```python
from build123d import *

# Parameters (mm, degrees)
SKETCH1_W            = 250
SKETCH1_H            = 90
BOSS_EXTRUDE1_DEPTH  = 4
SKETCH2_R            = 3
SKETCH2_R_2          = 1.5
SKETCH2_R_3          = 2
CUT_EXTRUDE1_DEPTH   = 133.91350571
SKETCH3_R            = 2
CUT_EXTRUDE2_DEPTH   = 133.91350571
CUT_EXTRUDE3_DEPTH   = 133.91350571
FILLET1_R            = 1
FILLET1_OF_MIRROR2_R = 1
MIRROR3_OUTLINE_R    = 1.5
MIRROR3_OUTLINE_R_2  = 2
MIRROR3_DEPTH        = 4


# Read off the part's stored shape, not the designer's step: Mirror3
with BuildPart() as part:
    # Sketch1 → Boss-Extrude1 (new body)
    with BuildSketch(Plane(origin=(0, 0, 0), x_dir=(0, 0, -1), z_dir=(1, 0, 0))):
        Rectangle(SKETCH1_W, SKETCH1_H)
    extrude(amount=BOSS_EXTRUDE1_DEPTH)

    # Sketch2 → Cut-Extrude1 (cut, through all)
    with BuildSketch(Plane(origin=(4, 0, 0), x_dir=(0, 0, -1), z_dir=(1, 0, 0))):
        Circle(SKETCH2_R)
        with Locations((-48, 0)):
            Circle(SKETCH2_R_2)
        with Locations((-89, 0)):
            Circle(SKETCH2_R_3)
        with Locations((-114, 0)):
            Circle(SKETCH2_R_2)
    extrude(amount=-CUT_EXTRUDE1_DEPTH, mode=Mode.SUBTRACT)

    # Sketch3 → Cut-Extrude2 (cut, through all)
    with BuildSketch(Plane(origin=(4, 0, 0), x_dir=(0, 0, -1), z_dir=(1, 0, 0))):
        with Locations((-20, 30)):
            Circle(SKETCH3_R)
    cut_extrude2 = extrude(amount=-CUT_EXTRUDE2_DEPTH, mode=Mode.SUBTRACT)

    # Sketch4 → Cut-Extrude3 (cut, through all)
    with BuildSketch(Plane(origin=(4, 0, 0), x_dir=(0, 0, -1), z_dir=(1, 0, 0))):
        with BuildLine():
            Line((-114, 7.5), (-50, 7.5))
            Line((-50, 7.5), (-42.5, 7.5))
            ThreePointArc((-42.5, 7.5), (-31.893398282, 11.893398282), (-27.5, 22.5))
            Line((-27.5, 22.5), (-27.5, 30))
            ThreePointArc((-27.5, 30), (-20, 37.5), (-12.5, 30))
            Line((-12.5, 30), (-12.5, 10))
            ThreePointArc((-12.5, 10), (-6.934403149, 14.427891494), (0, 16.007810594))
            Line((0, 16.007810594), (0, 45))
            Line((0, 45), (-125, 45))
            Line((-125, 45), (-125, 1.99556796))
            Line((-125, 1.99556796), (-125, 0))
            Line((-125, 0), (-121.5, 0))
            ThreePointArc((-121.5, 0), (-119.303300859, 5.303300859), (-114, 7.5))
        make_face()
    cut_extrude3 = extrude(amount=-CUT_EXTRUDE3_DEPTH, mode=Mode.SUBTRACT)

    # Fillet1
    fillet1_edges = [part.edges().sort_by_distance(p)[0] for p in [
        (2, 10, 12.5),
    ]]
    fillet(fillet1_edges, radius=FILLET1_R)

    # Mirror2: Cut-Extrude2, Cut-Extrude3 across plane
    add(cut_extrude2.mirror(Plane.ZX), mode=Mode.SUBTRACT)
    add(cut_extrude3.mirror(Plane.ZX), mode=Mode.SUBTRACT)

    # Fillet1 of Mirror2
    fillet1_of_mirror2_edges = [part.edges().sort_by_distance(p)[0] for p in [
        (2, -10, 12.5),
    ]]
    fillet(fillet1_of_mirror2_edges, radius=FILLET1_OF_MIRROR2_R)

    # Mirror3 outline → Mirror3 (cut)
    with BuildSketch(Plane.YZ):
        with BuildLine():
            Line((7.5, -42.5), (7.5, -114))
            ThreePointArc((7.5, -114), (0, -121.5), (-7.5, -114))
            Line((-7.5, -114), (-7.5, -42.5))
            ThreePointArc((-7.5, -42.5), (-11.893398282, -31.893398282), (-22.5, -27.5))
            Line((-22.5, -27.5), (-30, -27.5))
            ThreePointArc((-30, -27.5), (-37.5, -20), (-30, -12.5))
            Line((-30, -12.5), (-12.530587424, -12.5))
            ThreePointArc((-12.530587424, -12.5), (-11.615120349, -11.902392887), (-11.793832546, -10.823840071))
            ThreePointArc((-11.793832546, -10.823840071), (-14.917161888, -5.807605463), (-16.007810594, 0))
            Line((-16.007810594, 0), (-45, 0))
            Line((-45, 0), (-45, -125))
            Line((-45, -125), (45, -125))
            Line((45, -125), (45, 0))
            Line((45, 0), (16.007810594, 0))
            ThreePointArc((16.007810594, 0), (14.917161888, -5.807605463), (11.793832546, -10.823840071))
            ThreePointArc((11.793832546, -10.823840071), (11.615120349, -11.902392887), (12.530587424, -12.5))
            Line((12.530587424, -12.5), (30, -12.5))
            ThreePointArc((30, -12.5), (37.5, -20), (30, -27.5))
            Line((30, -27.5), (22.5, -27.5))
            ThreePointArc((22.5, -27.5), (11.893398282, -31.893398282), (7.5, -42.5))
        make_face()
        with Locations((0, -114)):
            Circle(MIRROR3_OUTLINE_R)
        with Locations((0, -89)):
            Circle(MIRROR3_OUTLINE_R_2)
        with Locations((0, -48)):
            Circle(MIRROR3_OUTLINE_R)
        with Locations((30, -20)):
            Circle(MIRROR3_OUTLINE_R_2)
        with Locations((-30, -20)):
            Circle(MIRROR3_OUTLINE_R_2)
    extrude(amount=MIRROR3_DEPTH, mode=Mode.SUBTRACT)


solid = part.part
```
Input: part model. Units: mm. Frame: model coordinates. A direction names the side the tool comes from. Round coordinates to 2 decimals unless told otherwise and drop trailing zeros. Write each loop counter-clockwise with the first axis right and the second up, starting at its lowest first coordinate (ties: lowest second). Pieces come first, ordered by that corner, then holes. Notation, with made-up numbers: (-39, 84.5) -> (1, 84.5) arc R10 ccw to (1, 95.5) -> close; hole circle Ø1 at (-16, 25.5). An arc over 180 degrees is marked (long way). Answer as CSV lines item,"result".
1. Contact query for flat-ended pins moving along their axis: P1, Ø5, axis at y = 30, z = -20, coming from the +X side; P2, Ø2, axis at x = 2, y = -25, coming from the +Z side; P3, Ø2, axis at x = 1.5, z = -85, coming from the -Y side; P4, Ø1.2, axis at x = 1.5, y = -26, coming from the -Z side. Output: stop coordinate, or through.
Geometry says:
P1,"stops at x = 4"
P2,"stops at z = 27.5"
P3,"stops at y = -7.5"
P4,"stops at z = -27.5"
2. Ray query, L1, parallel to Z at x = 0.5, y = -22.5; L2, parallel to Z at x = 3.1, y = 29; L3, parallel to Y at x = 2.25, z = -114. Return the intervals inside material, ascending. Write a range as [from, to].
Geometry says:
L1,"z = [-27.5, -12.5], [12.5, 27.5]"
L2,"z = [-27.5, -21.73], [-18.27, -12.5], [12.5, 18.27], [21.73, 27.5]"
L3,"y = [-7.5, -1.5], [1.5, 7.5]"
3. Reachability of faces 1 (the flat face through (2, -26, -27.5)), 2 (the flat face through (2, 7.5, 79)), 3 (the flat face through (2, -26, 27.5)), 4 (the flat face through (2, 26, -27.5)), 5 (the flat face through (2, 21, 12.5)) from +Z, -Z, +X, -X, +Y, -Y: full face, straight path, thin tool, end or side. Return the list, or none.
Geometry says:
face 1,"-Z, +X, -X, -Y"
face 2,"+Z, +X, -X, +Y"
face 3,"+Z, +X, -X, -Y"
face 4,"-Z, +X, -X, +Y"
face 5,"+X, -X, +Y"
4. Section A-A (x = 2.2). Give the number of separate pieces and of enclosed holes in the cut face, plus the area to 3 significant figures.
Geometry says:
separate pieces,"1"
enclosed holes,"11"
area,"5,700 mm^2"
5. Section C-C (z = -37.5). Return the cut outline in (x, y), plus the area to 3 significant figures.
Geometry says:
outline,"(0, -8.36) -> (4, -8.36) -> (4, 8.36) -> (0, 8.36) -> close"
area,"66.9 mm^2"
6. Mould query, pull axis Z, two halves, no side actions, for faces 6 (the flat face through (2, 7.5, -78)), 7 (the cylindrical face through (1.97, 0.16, -121.5)), 8 (the cylindrical face through (1.97, -37.5, -20.16)). Classes: +Z half, -Z half, draft (parallel to the pull), parting line (faces both ways), or undercut.
Geometry says:
face 6,"draft"
face 7,"-Z half"
face 8,"undercut"
7. Section B-B (z = 104.5). Return the cut outline in (x, y), plus the area to 3 significant figures.
Geometry says:
outline,"(0, -7.5) -> (4, -7.5) -> (4, 7.5) -> (0, 7.5) -> close"
area,"60.0 mm^2"
